Job drawing, mm, ordinate dimensions from the low corner. One solid piece. A direction names the side the tool comes from. Round coordinates to 2 decimals unless told otherwise and drop trailing zeros. Write each loop counter-clockwise with the first axis right and the second up, starting at its lowest first coordinate (ties: lowest second). Pieces come first, ordered by that corner, then holes. Notation, with made-up numbers: (50.5, 31.5) -> (97.5, 31.5) arc R23 cw to (97.5, 53.5) -> close; hole circle Ø8 at (71.5, 71). An arc over 180 degrees is marked (long way). Use CSV: the item, a comma, the result in double quotes. Start each with the question number.
(1) Saw through at D-D (y = 7.5). Give the cut face in (x, z) (1 decimal).
(2) Two-plate mould, pull along X, no slides. Class the marked faces 1, 2 and 3: released by +X, released by -X, zero draft, split by the parting line, or undercut.
(3) Saw through at B-B (x = 26). Give the cut face in (y, z).
(4) Drop flat-ended pins along their axis: pin 1 (4 mm diameter, centred on x = 28.5, z = 24, fed in from -Y); pin 2 (10 mm diameter, centred on x = 13.5, z = 14, fed in from -Y); pin 3 (6 mm diameter, centred on y = 11, z = 9, fed in from -X); pin 4 (4 mm diameter, centred on y = 6.5, z = 10.5, fed in from -X) (1 decimal). Give the stop position or say it passes through.
(5) Probe line 1 (X direction, y = 1, z = 10.25) (1 decimal); line 2 (Y direction, x = 51.5, z = 14.25); line 3 (Y direction, x = 11, z = 24.5). List the from-to ranges inside material, lowest first. Write a range as [from, to].
(6) Saw through at A-A (z = 5.75). Give the cut face in (x, y) (1 decimal).
(7) Saw through at C-C (z = 10). Give the cut face in (x, y) (1 decimal), plus the area to 3 significant figures.
(8) Which spindle directions (+Z, -Z, +X, -X, +Y, -Y) get a long thin tool onto all of the face, cutting with end or side? Do the marked faces 4 and 5. Say none if no direction does.
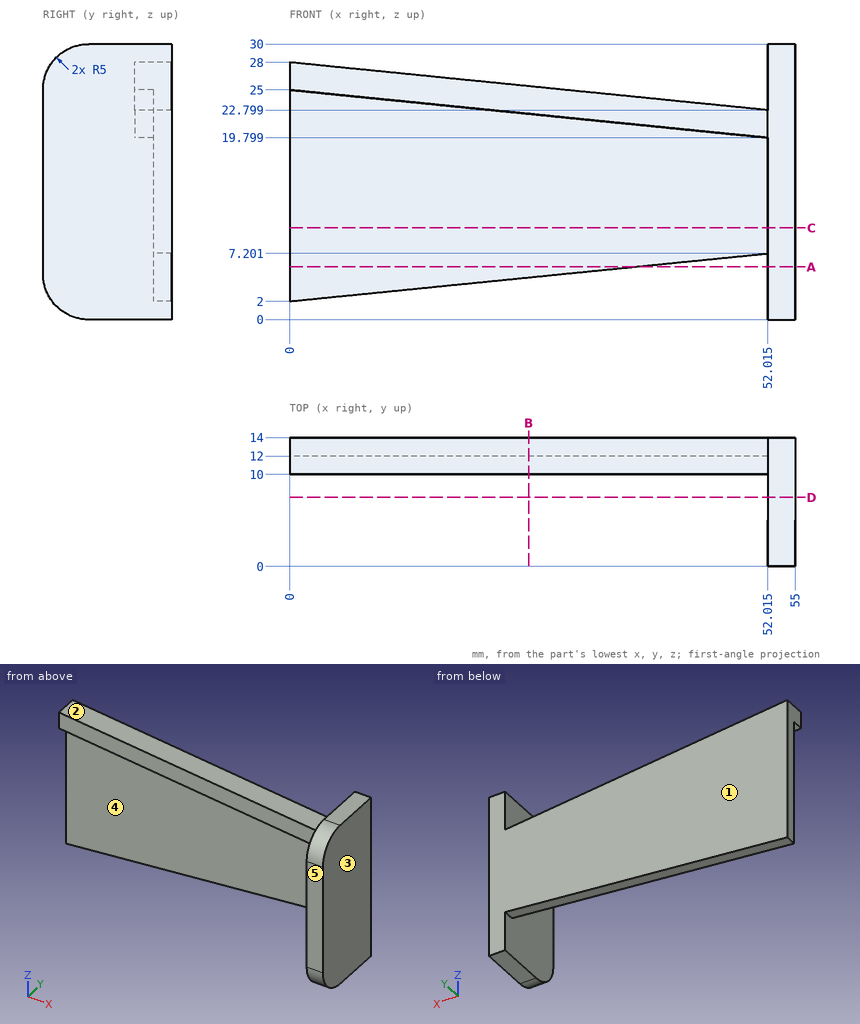
Answers:
1,outline,"(52, 0) -> (55, 0) -> (55, 30) -> (52, 30) -> close"
2,face 1,"zero draft"
2,face 2,"undercut"
2,face 3,"released by +X"
3,outline,"(10, 22.4) -> (12, 22.4) -> (12, 4.6) -> (14, 4.6) -> (14, 25.4) -> (10, 25.4) -> close"
4,pin 1,"stops at y = 10"
4,pin 2,"stops at y = 12"
4,pin 3,"stops at x = 0"
4,pin 4,"stops at x = 52"
5,line 1,"x = [52, 55]"
5,line 2,"y = [12, 14]"
5,line 3,"y = [10, 14]"
6,outline,"(0, 12) -> (37.5, 12) -> (37.5, 14) -> (0, 14) -> close; (52, 0) -> (55, 0) -> (55, 14) -> (52, 14) -> close"
7,outline,"(0, 12) -> (52, 12) -> (52, 0) -> (55, 0) -> (55, 14) -> (0, 14) -> close"
7,area,"146 mm²"
8,face 4,"-Z, -X, -Y"
8,face 5,"+Z, -Z, +X, -X, -Y"
